Build history of the part. All positions in model axes, mm. Face numbers are marked on the shaded views. A direction names the side the tool comes from. Round coordinates to 2 decimals unless told otherwise and drop trailing zeros. Order: outer loops, then holes, each group sorted by start corner. A loop starts at its lowest first (then second) coordinate and runs counter-clockwise, first axis right, second up. Notation, with made-up numbers: (-20.75, 25.25) -> (-11.75, 25.25) arc R32 ccw to (-11.75, 59.25) -> close; hole circle Ø11 at (3.5, 23). An arc over 180 degrees is marked (long way). Answer as a JSON object with one key per item and string values.
from build123d import *

# Parameters (mm, degrees)
F1_DEPTH = 21.5
F3_DEPTH = 19
F4_R     = 41
F5_DEPTH = 12
F6_R     = 5.7
F7_DEPTH = 43.001
F8_R     = 7.15
F9_DEPTH = 24.001


with BuildPart() as f1:
    # F0 (on Front) → F1 (new body, symmetric)
    with BuildSketch(Plane.XZ):
        with BuildLine():
            Line((-51.2549763874, 7), (-44.2549763874, 0))
            Line((-44.2549763874, 0), (-16.1883501321, 0))
            ThreePointArc((-16.1883501321, 0), (-12.923114351, -1.2134137678), (-11.2427113907, -4.2647058824))
            ThreePointArc((-11.2427113907, -4.2647058824), (-8.9058811875, -12.115672061), (-4.4669089907, -19))
            Line((-4.4669089907, -19), (0.7450236126, -19))
            Line((0.7450236126, -19), (29.7450236126, 14))
            Line((29.7450236126, 14), (29.7450236126, 33))
            Line((29.7450236126, 33), (24.7450236126, 38))
            Line((24.7450236126, 38), (5.7450236126, 38))
            ThreePointArc((5.7450236126, 38), (-3.7417667266, 29.8014254338), (-16.1883501321, 28.2853853987))
            Line((-16.1883501321, 28.2853853987), (-37.2549763874, 32))
            Line((-37.2549763874, 32), (-44.2549763874, 32))
            Line((-44.2549763874, 32), (-51.2549763874, 25))
            Line((-51.2549763874, 25), (-51.2549763874, 7))
        make_face()
    extrude(amount=F1_DEPTH, both=True)

    # F2 (on face) → F3 (cut)
    with BuildSketch(Plane.XZ.offset(21.5)):
        Polygon((-26.7216632598, 0), (-26.7216632598, 30.1426926993), (-37.2549763874, 32), (-44.2549763874, 32), (-51.2549763874, 25), (-51.2549763874, 7), (-44.2549763874, 0), align=None)
        with BuildLine():
            Line((17.4419933095, 0), (-16.1883501321, 0))
            ThreePointArc((-16.1883501321, 0), (-12.923114351, -1.2134137678), (-11.2427113907, -4.2647058824))
            ThreePointArc((-11.2427113907, -4.2647058824), (-8.9058811875, -12.115672061), (-4.4669089907, -19))
            Line((-4.4669089907, -19), (0.7450236126, -19))
            Line((0.7450236126, -19), (17.4419933095, 0))
        make_face()
    extrude(amount=-F3_DEPTH, mode=Mode.SUBTRACT)

    # F4 (on Front) → F5 (cut, symmetric)
    with BuildSketch(Plane.XZ):
        with Locations((24.7450236126, 41)):
            Circle(F4_R)
    extrude(amount=F5_DEPTH, both=True, mode=Mode.SUBTRACT)

    # F6 (on face) → F7 (cut, through all)
    with BuildSketch(Plane.XZ.offset(21.5)):
        with Locations((15.7450236126, 24)):
            Circle(F6_R)
    extrude(amount=-F7_DEPTH, mode=Mode.SUBTRACT)

    # F8 (on face) → F9 (cut, through all)
    with BuildSketch(Plane.XZ.offset(2.5)):
        with Locations((-37.2549763874, 14)):
            Circle(F8_R)
    extrude(amount=-F9_DEPTH, mode=Mode.SUBTRACT)


solid = f1.part
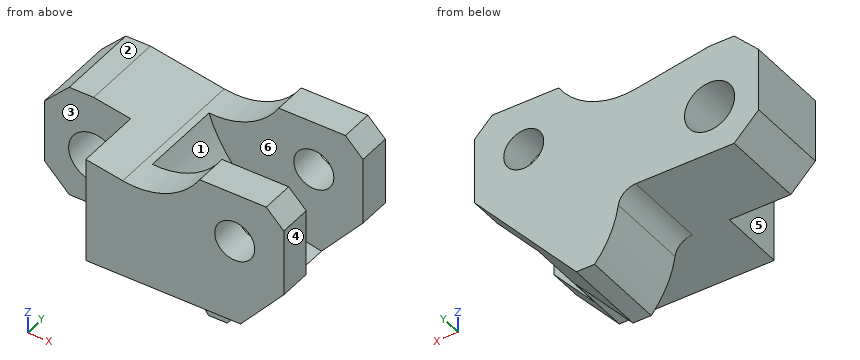
1) Cut at D-D, the plane z = 24. Give the cut face in (x, y), plus the area to 3 significant figures.
Checked values:
{"outline": "(-51.25, -2.5) -> (-26.72, -2.5) -> (-26.72, -21.5) -> (10.05, -21.5) -> (10.05, -12) -> (-12.56, -12) -> (-12.56, 12) -> (10.05, 12) -> (10.05, 21.5) -> (-51.25, 21.5) -> close; (21.45, -21.5) -> (29.75, -21.5) -> (29.75, -12) -> (21.45, -12) -> close; (21.45, 12) -> (29.75, 12) -> (29.75, 21.5) -> (21.45, 21.5) -> close", "area": "1,780 mm²"}
2) Cut at B-B, the plane y = -16. Give the cut face in (x, z), plus the area to 3 significant figures.
Checked values:
{"outline": "(-26.72, 0) -> (17.44, 0) -> (29.75, 14) -> (29.75, 33) -> (24.75, 38) -> (5.75, 38) arc R21.51 cw to (-16.19, 28.29) -> (-26.72, 30.14) -> close; hole circle Ø11.4 at (15.75, 24)", "area": "1,690 mm²"}
3) Flat gauge pins, fed straight in: pin 1 Ø13 at (x, y) = (-19, -10) entering from -Z; pin 2 Ø8 at (x, y) = (9.5, 2.5) entering from -Z; pin 3 Ø18 at (x, z) = (15.75, 24) entering from -Y; pin 4 Ø5.5 at (x, y) = (-40, 12.5) entering from +Z. Where does each tip first touch, or does it go through?
Checked values:
{"pin 1": "stops at z = 0", "pin 2": "stops at z = -13.59", "pin 3": "stops at y = -21.5", "pin 4": "stops at z = 32"}
4) Probe L1, parallel to Y at x = -28, z = 4.5; L2, parallel to X at y = -1, z = 20.5; L3, parallel to X at y = 1, z = 17. List the from-to ranges inside material, lowest first. Write a range as from..to.
Checked values:
{"L1": "y = -2.5..21.5", "L2": "x = -51.25..-40.23, -34.28..-10.76", "L3": "x = -51.25..-43.75, -30.76..-8.5"}
5) Cut at C-C, the plane x = 19. Give the cut face in (y, z), plus the area to 3 significant figures.
Checked values:
{"outline": "(-21.5, 1.77) -> (-12, 1.77) -> (-12, 19.32) -> (-21.5, 19.32) -> close; (-21.5, 28.68) -> (-12, 28.68) -> (-12, 38) -> (-21.5, 38) -> close; (12, 1.77) -> (21.5, 1.77) -> (21.5, 19.32) -> (12, 19.32) -> close; (12, 28.68) -> (21.5, 28.68) -> (21.5, 38) -> (12, 38) -> close", "area": "511 mm²"}
6) Cut at A-A, the plane y = 18. Give the cut face in (x, z).
Checked values:
{"outline": "(-51.25, 7) -> (-44.25, 0) -> (-16.19, 0) arc R5 cw to (-11.24, -4.26) arc R29 ccw to (-4.47, -19) -> (0.75, -19) -> (29.75, 14) -> (29.75, 33) -> (24.75, 38) -> (5.75, 38) arc R21.51 cw to (-16.19, 28.29) -> (-37.25, 32) -> (-44.25, 32) -> (-51.25, 25) -> close; hole circle Ø14.3 at (-37.25, 14); hole circle Ø11.4 at (15.75, 24)"}
7) Which spindle directions (+Z, -Z, +X, -X, +Y, -Y) get a long thin tool onto all of the face, cutting with end or side? Do the marked faces 4, 5 and 6. Say none if no direction does.
Checked values:
{"face 4": "+Z, -Z, +X, +Y, -Y", "face 5": "+Z, -Z, -X, -Y", "face 6": "+Z, +X"}
8) Pull direction Y, two halves, no side cores. Call the marked faces 1, 2 and 3: pulls with the +Y half, pulls with the -Y half, needs draft (parallel to the pull), parting line crosses it, or undercut.
Checked values:
{"face 1": "undercut", "face 2": "needs draft", "face 3": "pulls with the -Y half"}
